Autodesk Inventor part; units mm, degrees
ref_plane "Work Plane1" through (66.6877, 0, 0) normal (0, 0, -1) x (1, 0, 0)
ref_plane "YZ Plane" through (0, 0, 0) normal (1, 0, 0) x (0, 1, 0)
ref_plane "XZ Plane" through (0, 0, 0) normal (0, 1, 0) x (-1, 0, 0)
sketch "Sketch1" plane through (0, 0, 0) normal (0, 0, 1) x (1, 0, 0)
  line L0 (9.525, 0) -> (9.525, 1.5875)
  line L1 (9.525, 1.5875) -> (2.286, 1.5875)
  line L2 (0, 3.048) -> (0, 1.2192)
  line L3 (0, 1.2192) -> (1.5494, 1.2192)
  line L4 (1.5494, 1.2192) -> (2.2533, 0)
  line L5 (2.2533, 0) -> (9.525, 0)
  line L6 (0, 3.048) -> (0.6059, 3.048)
  line L7 (0.6059, 3.048) -> (2.286, 1.5875)
  line L8 (-1.905, 0) -> (11.43, 0)
  line L9 (0, -0.6096) -> (0, 3.6576)
  dimension "d0" = 9.525
  dimension "d1" = 1.5494
  dimension "d2" = 3.175
  dimension "d3" = 2.286
  dimension "d4" = 41
  dimension "d5" = 2.4384
  dimension "d6" = 60
  dimension "d7" = 6.096
revolve "Body" add sketch "Sketch1" angle 360 about axis through (2.2533, 0, 0) along (1, 0, 0) contours L5 L4 L3 L2 L6 L7 L1 L0
sketch "Sketch2" plane through (0, 0, 0) normal (-1, 0, 0) x (0, 0, 1)
  circle A0 centre (0, 0) radius 3.048
  circle A1 centre (0, 0) radius 1.2192
  line L0 (0.9421, 0.2524) -> (1.1777, 0.3156)
  line L1 (0.9421, -0.2524) -> (1.1777, -0.3156)
  arc A2 (0.9421, -0.2524) -> (0.9421, 0.2524) centre (0, 0) ccw
  arc A3 (1.1777, -0.3156) -> (1.1777, 0.3156) centre (0, 0) ccw
  line L2 (0, -4.2672) -> (0, 4.2672)
  line L3 (-4.2672, 0) -> (4.2672, 0)
  line L4 (0.9421, 0.2524) -> (0, 0) construction
  line L5 (0, 0) -> (0.9421, -0.2524) construction
  line L6 (0.2524, 0.9421) -> (0.3156, 1.1777)
  line L7 (0.6897, 0.6897) -> (0.8621, 0.8621)
  arc A4 (0.6897, 0.6897) -> (0.2524, 0.9421) centre (0, 0) ccw
  arc A5 (0.8621, 0.8621) -> (0.3156, 1.1777) centre (0, 0) ccw
  line L8 (-0.6897, 0.6897) -> (-0.8621, 0.8621)
  line L9 (-0.2524, 0.9421) -> (-0.3156, 1.1777)
  arc A6 (-0.2524, 0.9421) -> (-0.6897, 0.6897) centre (0, 0) ccw
  arc A7 (-0.3156, 1.1777) -> (-0.8621, 0.8621) centre (0, 0) ccw
  line L10 (-0.9421, -0.2524) -> (-1.1777, -0.3156)
  line L11 (-0.9421, 0.2524) -> (-1.1777, 0.3156)
  arc A8 (-0.9421, 0.2524) -> (-0.9421, -0.2524) centre (0, 0) ccw
  arc A9 (-1.1777, 0.3156) -> (-1.1777, -0.3156) centre (0, 0) ccw
  line L12 (-0.2524, -0.9421) -> (-0.3156, -1.1777)
  line L13 (-0.6897, -0.6897) -> (-0.8621, -0.8621)
  arc A10 (-0.6897, -0.6897) -> (-0.2524, -0.9421) centre (0, 0) ccw
  arc A11 (-0.8621, -0.8621) -> (-0.3156, -1.1777) centre (0, 0) ccw
  line L14 (0.6897, -0.6897) -> (0.8621, -0.8621)
  line L15 (0.2524, -0.9421) -> (0.3156, -1.1777)
  arc A12 (0.2524, -0.9421) -> (0.6897, -0.6897) centre (0, 0) ccw
  arc A13 (0.3156, -1.1777) -> (0.8621, -0.8621) centre (0, 0) ccw
  dimension "d8" = 1.9507
  dimension "d9" = 2.4384
  dimension "d10" = 15
  dimension "d11" = 15
  dimension "d22" = 360
extrude "Slot" add sketch "Sketch2" against normal up to next contours L3 A2 L0 A1 | A1 L1 A2 L3 | L3 A8 L10 A1 | A1 L11 A8 L3 | A1 L7 A4 L6 | L9 A6 L8 A1 | A1 L13 A10 L12 | L15 A12 L14 A1
thread "Thread"
chamfer "Chamfer1" distance 0.3785 distance2 0.7569 1 edges at (9.525, -1.5875, 0) measured on face at (9.525, -0.1593, -0.6099)
ref_plane "Work Plane1" through (66.6877, 0, 0) normal (0, 0, -1) x (1, 0, 0)
equation "\"d0\" = NLG"
equation "\"d1\" = INTI"
equation "\"d2\" = GD"
equation "\"d3\" = KOH"
equation "\"d4\" = 0.5 * SEWI"
equation "\"d5\" = SW"
equation "\"d7\" = KOD"
equation "\"d8\" = 0.8 * SW"
equation "\"d9\" = SW"
equation "\"d15\" = GEL"
equation "\"d17\" = -0.5 * SPD + 0.5 * GD"
equation "\"d18\" = GUL"
equation "\"NLG\" = 9.525"
equation "\"SW\" = 2.4384"
equation "\"INTI\" = 1.5494"
equation "\"GEL\" = 5.6515"
equation "\"KOH\" = 2.286"
equation "\"KOD\" = 6.096"
equation "\"GUL\" = 0.75692"
equation "\"SPD\" = 2.41808"
equation "\"GD\" = NND"
equation "\"SEWI\" = 82deg"
equation "\"TOA\" = 30deg"
equation "\"GD1\" = SPD"
equation "\"EPV\" = 4.11221"
equation "\"THREADDIA\" = 3.175"
equation "\"BDM\" = NND"
equation "\"NND\" = 3.175"
equation "\"GAL\" = 1.5875"
equation "\"E0\" = 1.155 * SW"
properties part number "ANSI B18.3 - 5-40 UNC x 0.375, SSFCHCSI" material "Steel, Mild"
Design review of the part built by this model. Coordinates are the model's own, in mm. Give positions to 0.01 mm unless a question says otherwise; leave off trailing zeros. Order: outer loops, then holes, each group sorted by start corner. A loop starts at its lowest first (then second) coordinate and runs counter-clockwise, first axis right, second up. Notation, with made-up numbers: (27.5, 79.5) -> (40.5, 79.5) arc R25 cw to (40.5, 102.5) -> close; hole circle Ø11 at (8.25, -40). An arc over 180 degrees is marked (long way). Write item = value, one per line. Start each with the question number.
(1) For pin 1 (3 mm diameter, centred on x = 4.5, z = 2.5, fed in from +Y), flat-tipped, find the tip position at first contact; note if it passes through.
(2) We need section A-A on x = 7.25. Write out the cut boundary in (y, z) (1 decimal).
(3) To check wall thickness, follow line 1 along Z through (x, y) = (0.5, 0); line 2 along Z through (x, y) = (8.25, 0); line 3 along Y through (x, z) = (8.5, 1.25). State the ranges of each line that lie inside material, in increasing order.
(4) We need section B-B on x = 2. Write out the cut boundary in (y, z), plus the area to 3 significant figures.
(5) Mouldability with a two-part tool opening along Y and no side actions: class faces 1 (the face through (9.525, 0, 0)), 2 (the face through (2.21, 0.07, -0.02)), 3 (the face through (5.48, -0.34, 1.55)) as +Y half, -Y half, draft (parallel to the pull), parting line (faces both ways), or undercut.
Numbers:
q1.pin_1 = 1.23
q2.outline = circle Ø3.2 at (0, 0)
q3.line_1 = -3.05 to -0.98, 0.98 to 3.05
q3.line_2 = -1.59 to 1.59
q3.line_3 = -0.98 to 0.98
q4.outline = circle Ø3.67 at (0, 0); hole circle Ø0.88 at (0, 0)
q4.area = 9.99 mm^2
q5.face_1 = draft
q5.face_2 = undercut
q5.face_3 = parting line
